The model under review builds one solid part; all positions refer to its coordinate system, in mm. Face numbers are marked on the shaded views. Round coordinates to 2 decimals unless told otherwise and drop trailing zeros. Write each loop counter-clockwise with the first axis right and the second up, starting at its lowest first coordinate (ties: lowest second). Pieces come first, ordered by that corner, then holes.
Item 1: Add section B-B (y = 0). Give the boundary of the cut face in (x, z).
Item 2: To check wall thickness, follow L1, parallel to Z at x = -4, y = -10; L2, parallel to Z at x = -10, y = 4.5; L3, parallel to X at y = 0, z = 12. State the ranges of each line that lie inside material, in increasing order.
Item 3: Add section D-D (z = 13.5). Give the boundary of the cut face in (x, y), plus the area to 3 significant figures.
Item 4: Draft analysis for pull direction Y (two halves, no side actions). For the marked faces 1, 2, 3 and 4, state which applies: +Y half, -Y half, draft (parallel to the pull), parting line (faces both ways), or undercut.
Item 5: Add section A-A (z = 0). Give the boundary of the cut face in (x, y).
Item 6: Add section C-C (x = 0). Give the boundary of the cut face in (y, z).
Item 7: Clearance check with flat-ended pins moving along their axes: pin 1 Ø2 at (y, z) = (-4.5, -15) entering from -X; pin 2 Ø1.5 at (y, z) = (8, -5) entering from -X; pin 3 Ø12 at (x, z) = (-4, -6) entering from -Y; pin 4 Ø10 at (y, z) = (-4.5, -8) entering from -X. State where each tip first meets the part, or that it passes through.
```python
from build123d import *

# Parameters (mm, degrees)
SKETCH1_W               = 10
SKETCH1_H               = 50
SKETCH2_W               = 30
SKETCH2_H               = 6
CUT_EXTRUDE1_DEPTH      = 12.7
CUT_EXTRUDE1_DEPTH_BACK = 12.7
SKETCH3_W               = 1.6
SKETCH3_H               = 21.427389106
SKETCH3_3_W             = 1.6
SKETCH3_3_H             = 21.427389106


with BuildPart() as part:
    # Sketch1 → Revolve1 (revolve)
    with BuildSketch(Plane(origin=(0, 0, 0), x_dir=(1, 0, 0), z_dir=(0, 1, 0))):
        with Locations((10, 0)):
            Rectangle(SKETCH1_W, SKETCH1_H)
    revolve(axis=Axis((0, 0, 25), (0, 0, -1)))

    # Sketch2 → Cut-Extrude1 (cut, two sides)
    with BuildSketch(Plane.XY) as cut_extrude1_sk:
        with Locations((0, -12)):
            Rectangle(SKETCH2_W, SKETCH2_H)
    extrude(amount=CUT_EXTRUDE1_DEPTH, mode=Mode.SUBTRACT)
    extrude(cut_extrude1_sk.sketch, amount=-CUT_EXTRUDE1_DEPTH_BACK, mode=Mode.SUBTRACT)

    # Sketch3 → Cut-Revolve1 (revolve, cut)
    with BuildSketch(Plane.XY):
        with Locations((9.2, 1.713694553)):
            Rectangle(SKETCH3_W, SKETCH3_H)
    revolve(axis=Axis((10, -9, 0), (0, -1, 0)), mode=Mode.SUBTRACT)

    # Sketch3_3 → Cut-Revolve2 (revolve, cut)
    with BuildSketch(Plane.XY):
        with Locations((-9.2, 1.713694553)):
            Rectangle(SKETCH3_3_W, SKETCH3_3_H)
    revolve(axis=Axis((-10, -9, 0), (0, -1, 0)), mode=Mode.SUBTRACT)


solid = part.part
```
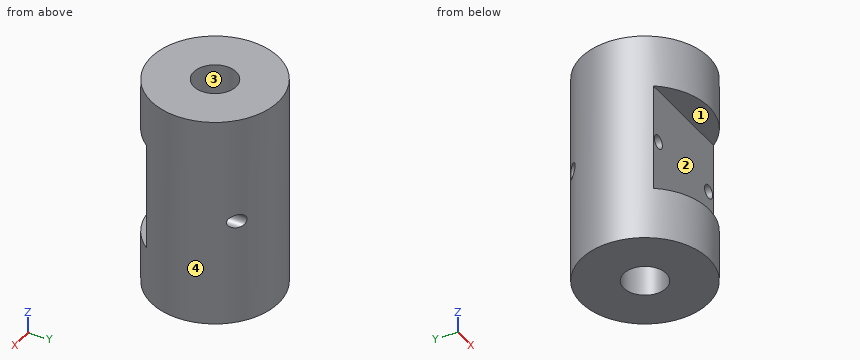
Numbers:
1. outline: (-15, -25) - (-5, -25) - (-5, 25) - (-15, 25) - close; (5, -25) - (15, -25) - (15, 25) - (5, 25) - close; hole circle Ø3.2 at (-10, 0); hole circle Ø3.2 at (10, 0)
2. L1: z = -25 to -12.7, 12.7 to 25
2. L2: z = -25 to -1.6, 1.6 to 25
2. L3: x = -15 to -5, 5 to 15
3. outline: circle Ø30 at (0, 0); hole circle Ø10 at (0, 0)
3. area: 628 mm2
4. face 1: draft
4. face 2: -Y half
4. face 3: undercut
4. face 4: parting line
5. outline: (-12, -9) - (-11.6, -9) - (-11.6, 9.51) arc R15 ccw to start; (-8.4, -9) - (8.4, -9) - (8.4, 12.43) arc R15 ccw to (-8.4, 12.43) - close; (11.6, -9) - (12, -9) arc R15 ccw to (11.6, 9.51) - close; hole circle Ø10 at (0, 0)
6. outline: (-15, -25) - (-5, -25) - (-5, 25) - (-15, 25) - (-15, 12.7) - (-9, 12.7) - (-9, -12.7) - (-15, -12.7) - close; (5, -25) - (15, -25) - (15, 25) - (5, 25) - close
7. pin 1: stops at x = -14.59
7. pin 2: stops at x = -13.13
7. pin 3: stops at y = -9
7. pin 4: stops at x = -15
